Check sheet for the modelled part. Datum: model origin and axes. Units: mm. Face numbers are marked on the shaded views. A direction names the side the tool comes from. Coordinates: 2 decimals unless noted, no trailing zeros. Write each loop counter-clockwise with the first axis right and the second up, starting at its lowest first coordinate (ties: lowest second). Pieces come first, ordered by that corner, then holes. Notation, with made-up numbers: (38.25, 10) - (59.25, 10) arc R16 cw to (59.25, 33) - close; hole circle Ø2 at (-37, 58). An arc over 180 degrees is marked (long way). Use one line per item in the form item = value. Start each with the question number.
1. Cross-section at B-B on y = 18. Record the boundary of the cut face in (x, z).
2. Go/stop test with flat-tipped pins: pin 1 Ø3 at (y, z) = (44, -24.5) entering from -X; pin 2 Ø22 at (y, z) = (29.5, -15.5) entering from +X; pin 3 Ø3 at (y, z) = (14, -34.5) entering from +X; pin 4 Ø8 at (x, z) = (47, -36.5) entering from -Y. Record where each tip stops, or that it passes through.
3. Draft check along Z on the marked faces 4, 5 and 6. Enter one of: +Z half, -Z half, draft (parallel to the pull), parting line (faces both ways), or undercut.
4. Cross-section at C-C on z = -15. Record the boundary of the cut face in (x, y), then the cut area to 3 significant figures.
5. Scan lines: line 1 along Z through (x, y) = (3, 25); line 2 along X through (y, z) = (30.5, -15.5); line 3 along Z through (x, y) = (14, 45). Record each from-to range of solid material in increasing order.
6. Tool access check on the marked faces 1, 2 and 3. Record the directions out of +Z, -Z, +X, -X, +Y, -Y that give a thin tool (end or side, any length) a straight path to the whole face; none if there is none.
7. Cross-section at A-A on x = 8.5. Record the boundary of the cut face in (y, z).
8. Cross-section at D-D on x = 35. Record the boundary of the cut face in (y, z).
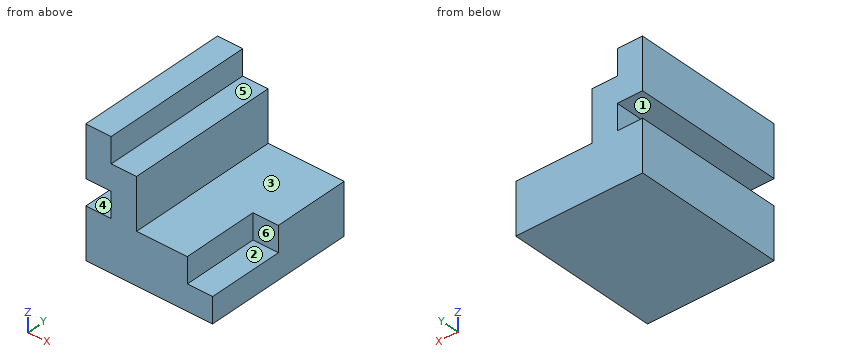
Autodesk Inventor part; units mm, degrees
ref_plane "YZ Plane" through (0, 0, 0) normal (1, 0, 0) x (0, 1, 0)
ref_plane "XZ Plane" through (0, 0, 0) normal (0, 1, 0) x (-1, 0, 0)
ref_plane "XY Plane" through (0, 0, 0) normal (0, 0, 1) x (1, 0, 0)
sketch "Náčrt1" plane through (0, 0, 0) normal (1, 0, 0) x (0, 1, 0)
  line L0 (0, 0) -> (0, -50)
  line L1 (0, -50) -> (60, -50)
  line L2 (60, -50) -> (60, 0)
  line L3 (60, 0) -> (0, 0)
  dimension "d0" = 50
  dimension "d1" = 60
extrude "Vysunutí1" add sketch "Náčrt1" along normal blind 50
sketch "Náčrt2" plane through (50, 0, 0) normal (1, 0, 0) x (0, 0, -1)
  line L0 (50, 0) -> (50, 60)
  line L1 (50, 60) -> (50, 30)
  line L2 (50, 30) -> (40, 30)
  line L3 (40, 30) -> (40, 0)
  line L4 (0, 0) -> (50, 0)
  line L5 (40, 0) -> (30, 0)
  line L6 (30, 0) -> (30, 30)
  line L7 (30, 30) -> (40, 30)
  dimension "d4" = 30
  dimension "d5" = 10
  dimension "d6" = 10
extrude "Vysunutí2" cut sketch "Náčrt2" against normal blind 10 contours L4 L6 L7 L3
sketch "Náčrt3" plane through (50, 0, 0) normal (1, 0, 0) x (0, 0, -1)
  point P0 (0, 0)
sketch "Náčrt4" plane through (50, 0, 0) normal (1, 0, 0) x (0, 0, -1)
  line L0 (0, 0) -> (30, 0)
  line L1 (0, 0) -> (30, 0)
  line L2 (30, 0) -> (30, 60)
  line L3 (50, 60) -> (0, 60)
  line L4 (0, 60) -> (0, 0)
  line L5 (30, 60) -> (0, 60)
  line L6 (0, 60) -> (0, 0)
  dimension "d9" = 30
extrude "Vysunutí3" cut sketch "Náčrt4" against normal blind 30
sketch "Náčrt5" plane through (20, 0, 0) normal (1, 0, 0) x (0, 0, -1)
  line L0 (30, 0) -> (0, 0)
  line L1 (0, 0) -> (10, 0)
  line L2 (10, 0) -> (10, 60)
  line L3 (50, 60) -> (0, 60)
  line L4 (0, 60) -> (0, 0)
  line L5 (0, 60) -> (10, 60)
  line L6 (0, 60) -> (0, 0)
  dimension "d12" = 10
extrude "Vysunutí4" cut sketch "Náčrt5" against normal blind 10
sketch "Náčrt6" plane through (0, 0, 0) normal (-1, 0, 0) x (0, 0, 1)
  line L0 (-50, 60) -> (0, 60)
  line L1 (0, 60) -> (-20, 60)
  line L2 (-30, 60) -> (-30, 30)
  line L3 (-20, 60) -> (-30, 60)
  line L4 (-30, 0) -> (-30, 30)
  line L5 (-30, 60) -> (-30, 0)
  line L6 (-30, 0) -> (-20, 0)
  line L7 (-30, 0) -> (-10, 0)
  line L8 (-20, 0) -> (-20, 60)
  point P0 (0, 0)
  dimension "d15" = 20
  dimension "d16" = 10
extrude "Vysunutí5" cut sketch "Náčrt6" against normal blind 10
properties part number "Martin-Probst-26673_obrazek_3"
Final values:
q1.outline = (0, -50) - (50, -50) - (50, -40) - (40, -40) - (40, -30) - (20, -30) - (20, -10) - (10, -10) - (10, 0) - (0, 0) - (0, -20) - (10, -20) - (10, -30) - (0, -30) - close
q2.pin_1 = 10
q2.pin_2 = 20
q2.pin_3 = 40
q2.pin_4 = 0
q3.face_4 = undercut
q3.face_5 = +Z half
q3.face_6 = draft
q4.outline = (0, 0) - (20, 0) - (20, 60) - (0, 60) - close
q4.area = 1,200 mm²
q5.line_1 = -50 to -30, -20 to 0
q5.line_2 = 0 to 20
q5.line_3 = -50 to -10
q6.face_1 = -X, +Y, -Y
q6.face_2 = +Z, +X, -Y
q6.face_3 = +Z, +X, +Y, -Y
q7.outline = (0, -50) - (60, -50) - (60, -30) - (0, -30) - close; (0, -20) - (60, -20) - (60, 0) - (0, 0) - close
q8.outline = (0, -50) - (60, -50) - (60, -30) - (0, -30) - close
